from build123d import *

# Parameters (mm, degrees)
EXTRUDE_1_DEPTH     = 5
SKETCH_3_R          = 1.5
CUT_EXTRUDE_1_DEPTH = 114.61053585


with BuildPart() as part:
    # 草图1 → 凸台-拉伸1 (new body)
    with BuildSketch(Plane(origin=(0, 0, 0), x_dir=(1, 0, 0), z_dir=(0, 1, 0))):
        with BuildLine():
            Line((-25.929831279, 46.15942029), (34.070168721, 46.15942029))
            ThreePointArc((34.070168721, 46.15942029), (37.605702627, 44.694954196), (39.070168721, 41.15942029))
            Line((39.070168721, 41.15942029), (39.070168721, -8.84057971))
            Line((39.070168721, -8.84057971), (43.820168721, -8.84057971))
            ThreePointArc((43.820168721, -8.84057971), (45.234382283, -9.426366148), (45.820168721, -10.84057971))
            Line((45.820168721, -10.84057971), (45.820168721, -46.84057971))
            ThreePointArc((45.820168721, -46.84057971), (45.234382283, -48.254793273), (43.820168721, -48.84057971))
            Line((43.820168721, -48.84057971), (39.070168721, -48.84057971))
            Line((39.070168721, -48.84057971), (39.070168721, -98.84057971))
            ThreePointArc((39.070168721, -98.84057971), (37.605702627, -102.376113616), (34.070168721, -103.84057971))
            Line((34.070168721, -103.84057971), (-25.929831279, -103.84057971))
            ThreePointArc((-25.929831279, -103.84057971), (-29.465365185, -102.376113616), (-30.929831279, -98.84057971))
            Line((-30.929831279, -98.84057971), (-30.929831279, -48.84057971))
            Line((-30.929831279, -48.84057971), (-35.679831279, -48.84057971))
            ThreePointArc((-35.679831279, -48.84057971), (-37.094044841, -48.254793273), (-37.679831279, -46.84057971))
            Line((-37.679831279, -46.84057971), (-37.679831279, -10.84057971))
            ThreePointArc((-37.679831279, -10.84057971), (-37.094044841, -9.426366148), (-35.679831279, -8.84057971))
            Line((-35.679831279, -8.84057971), (-30.929831279, -8.84057971))
            Line((-30.929831279, -8.84057971), (-30.929831279, 41.15942029))
            ThreePointArc((-30.929831279, 41.15942029), (-29.465365185, 44.694954196), (-25.929831279, 46.15942029))
        make_face()
    extrude(amount=EXTRUDE_1_DEPTH)

    # 草图3 → 切除-拉伸1 (cut, through all)
    with BuildSketch(Plane(origin=(0, 5, 0), x_dir=(1, 0, 0), z_dir=(0, 1, 0))):
        with Locations(Location((34.070168721, 41.15942029, 0), (0, 0, 270))):
            Circle(SKETCH_3_R)
        with Locations(Location((-25.929831279, 41.15942029, 0), (0, 0, 270))):
            Circle(SKETCH_3_R)
        with Locations(Location((-25.929831279, -98.84057971, 0), (0, 0, 270))):
            Circle(SKETCH_3_R)
        with Locations(Location((34.070168721, -98.84057971, 0), (0, 0, 270))):
            Circle(SKETCH_3_R)
        with Locations(Location((34.070168721, -28.84057971, 0), (0, 0, 270))):
            Circle(SKETCH_3_R)
        with Locations(Location((-25.929831279, -28.84057971, 0), (0, 0, 270))):
            Circle(SKETCH_3_R)
    extrude(amount=-CUT_EXTRUDE_1_DEPTH, mode=Mode.SUBTRACT)


solid = part.part
Read the model definition and answer for the solid it produces. Units are mm, in the model's axes. A direction names the side the tool comes from. Give positions to 0.01 mm unless a question says otherwise; leave off trailing zeros. Write each loop counter-clockwise with the first axis right and the second up, starting at its lowest first coordinate (ties: lowest second). Pieces come first, ordered by that corner, then holes. Notation, with made-up numbers: (-20, -19.75) -> (4, -19.75) arc R20 cw to (4, -6.75) -> close; hole circle Ø6 at (79, 18). An arc over 180 degrees is marked (long way). Answer as a JSON object with one key per item and string values. Group by question number.
1) Find section A-A (y = 1.3). Write down the section's boundary in (x, z).
2) Consider L1, parallel to Z at x = -26, y = 4; L2, parallel to X at y = 0.8, z = 97.5; L3, parallel to X at y = 0.7, z = 50.5. Determine where each line is inside the solid, lowest interval first. Write a range as from..to.
3) Find section B-B (z = 67.5). Write down the section's boundary in (x, y).
4) A tool of negligible diameter and unlimited length cuts with its end or side. For faces 4 (the flat face through (-33, 2, 8.841)), 5 (the flat face through (39.07, 2, -17)), 6 (the flat face through (39.07, 2, 73)), 7 (the flat face through (-30.93, 2, 74)), from which of +Z, -Z, +X, -X, +Y, -Y can it reach the whole face along a straight path? Write none if from no direction.
5) The mould has two halves that part along X. Classify faces 1 (the cylindrical face through (-29.5, 2.46, -44.66)), 2 (the flat face through (5, 0, 28)), 3 (the cylindrical face through (-26.5, 2.54, 100.23)): +X half, -X half, draft (parallel to the pull), parting line (faces both ways), or undercut.
6) Each of these flat-tipped pins is pushed along its axis until it touches: P1, Ø2.5, axis at y = 2, z = 83, coming from the +X side; P2, Ø2.5, axis at y = 3.5, z = -18, coming from the -X side; P3, Ø2.5, axis at x = -33.5, y = 2.5, coming from the +Z side. Where does it stop, or does it pass through?
Values follow:
{
 "1": {"outline": "(-37.68, 10.84) arc R2 ccw to (-35.68, 8.84) -> (-30.93, 8.84) -> (-30.93, -41.16) arc R5 ccw to (-25.93, -46.16) -> (34.07, -46.16) arc R5 ccw to (39.07, -41.16) -> (39.07, 8.84) -> (43.82, 8.84) arc R2 ccw to (45.82, 10.84) -> (45.82, 46.84) arc R2 ccw to (43.82, 48.84) -> (39.07, 48.84) -> (39.07, 98.84) arc R5 ccw to (34.07, 103.84) -> (-25.93, 103.84) arc R5 ccw to (-30.93, 98.84) -> (-30.93, 48.84) -> (-35.68, 48.84) arc R2 ccw to (-37.68, 46.84) -> close; hole circle Ø3 at (-25.93, -41.16); hole circle Ø3 at (-25.93, 28.84); hole circle Ø3 at (-25.93, 98.84); hole circle Ø3 at (34.07, -41.16); hole circle Ø3 at (34.07, 28.84); hole circle Ø3 at (34.07, 98.84)"},
 "2": {"L1": "z = -46.16..-42.66, -39.66..27.34, 30.34..97.34, 100.34..103.84", "L2": "x = -30.93..-26.6, -25.26..33.4, 34.74..39.07", "L3": "x = -30.93..39.07"},
 "3": {"outline": "(-30.93, 0) -> (39.07, 0) -> (39.07, 5) -> (-30.93, 5) -> close"},
 "4": {"face 4": "-Z, -X, +Y, -Y", "face 5": "-Z, +X, +Y, -Y", "face 6": "+Z, +X, +Y, -Y", "face 7": "+Z, -X, +Y, -Y"},
 "5": {"face 1": "-X half", "face 2": "draft", "face 3": "undercut"},
 "6": {"P1": "stops at x = 39.07", "P2": "stops at x = -30.93", "P3": "stops at z = 48.84"}
}
